Source: CAD feature listing. Evaluate the final solid. Frame: model axes, mm. A direction names the side the tool comes from. Round coordinates to 2 decimals unless told otherwise and drop trailing zeros. Order: outer loops, then holes, each group sorted by start corner. A loop starts at its lowest first (then second) coordinate and runs counter-clockwise, first axis right, second up.
Autodesk Inventor part; units mm, degrees
ref_plane "YZ Plane" through (0, 0, 0) normal (1, 0, 0) x (0, 1, 0)
ref_plane "XZ Plane" through (0, 0, 0) normal (0, 1, 0) x (-1, 0, 0)
ref_plane "XY Plane" through (0, 0, 0) normal (0, 0, 1) x (1, 0, 0)
sketch "Sketch1" plane through (0, 0, 0) normal (0, 1, 0) x (-1, 0, 0)
  line L0 (100, -50) -> (-100, -50)
  line L1 (-100, -50) -> (-100, 50)
  line L2 (-100, 50) -> (100, 50)
  line L3 (100, 50) -> (100, -50)
  line L4 (100, -50) -> (-100, 50) construction
  line L5 (-100, -50) -> (100, 50) construction
  line L6 (-40, -30) -> (-80, -30)
  line L7 (-50, -50) -> (-70, -50)
  line L8 (-40, -30) -> (-50, -50)
  line L9 (-80, -30) -> (-70, -50)
  line L10 (80, -30) -> (40, -30)
  line L11 (70, -50) -> (50, -50)
  line L12 (80, -30) -> (70, -50)
  line L13 (40, -30) -> (50, -50)
  line L14 (-100, -10) -> (-100, 10)
  line L15 (-80, -20) -> (-80, 20)
  line L16 (-80, -20) -> (-100, -10)
  line L17 (-80, 20) -> (-100, 10)
  line L18 (100, -50) -> (-100, -50)
  line L19 (-100, -50) -> (-100, -80)
  line L20 (-100, -80) -> (100, -80)
  line L21 (100, -80) -> (100, -50)
  line L22 (-40, -70) -> (-80, -70)
  line L23 (-40, -70) -> (-50, -50)
  line L24 (-80, -70) -> (-70, -50)
  line L25 (80, -70) -> (40, -70)
  line L26 (80, -70) -> (70, -50)
  line L27 (40, -70) -> (50, -50)
  line L28 (-100, -80) -> (-200, -80)
  line L29 (-200, -80) -> (-200, -50)
  line L30 (-200, -50) -> (-100, -50)
  line L31 (-100, -50) -> (-100, -80)
  line L32 (-160, -70) -> (-150, -50)
  line L33 (-160, -70) -> (-120, -70)
  line L34 (-120, -70) -> (-130, -50)
  line L35 (0, -80) -> (0, -50)
  point P0 (0, 0)
  point P1 (-100, 10)
  point P2 (-100, -10)
  point P3 (-70, -50)
  point P4 (-50, -50)
  point P5 (70, -50)
  point P6 (0, 0)
  point P7 (0, 0)
  point P8 (-100, -50)
  point P9 (-100, -50)
  point P10 (-100, -50)
  dimension "d72" = 200
  dimension "d73" = 100
  dimension "d78" = 20
  dimension "d79" = 40
  dimension "d80" = 20
  dimension "d81" = 10
  dimension "d82" = 20
  dimension "d83" = 40
  dimension "d84" = 20
  dimension "d85" = 10
  dimension "d86" = 120
  dimension "d87" = 30
  dimension "d88" = 0
  dimension "d89" = 0
  dimension "d90" = 40
  dimension "d91" = 20
  dimension "d92" = 20
  dimension "d93" = 10
  dimension "d94" = 40
  dimension "d95" = 0
  dimension "d114" = 200
  dimension "d115" = 30
  dimension "d128" = 100
sketch "Sketch1 outline for Extrusion28" plane through (0, 0, 0) normal (0, 1, 0) x (-1, 0, 0)
  line L0 (-200, -50) -> (-200, -80)
  line L1 (-100, -50) -> (-200, -50)
  line L2 (-100, -80) -> (-100, -50)
  line L3 (-200, -80) -> (-100, -80)
extrude "Extrusion28" add sketch "Sketch1 outline for Extrusion28" along normal blind 12
sketch "Sketch1 outline for Extrusion29" plane through (0, 0, 0) normal (0, 1, 0) x (-1, 0, 0)
  line L0 (-160, -70) -> (-120, -70)
  line L1 (-150, -50) -> (-160, -70)
  line L2 (-130, -50) -> (-150, -50)
  line L3 (-120, -70) -> (-130, -50)
extrude "Extrusion29" cut sketch "Sketch1 outline for Extrusion29" along normal blind 6
fillet "Fillet17" radius 6 2 edges at (150, 0, -80) (150, 12, -80)
fillet "Fillet18" radius 2 2 edges at (120, 3, -70) (160, 3, -70)
fillet "Fillet19" radius 1 5 edges at (158.4652, 0, -69.0515) (140, 0, -70) (121.5348, 0, -69.0515) (125.7236, 0, -58.5528) (154.2764, 0, -58.5528)
mirror "Mirror1" about plane through (100, 0, -80) normal (-1, 0, 0) of "Extrusion28", "Fillet17", "Extrusion29", "Fillet18", "Fillet19"
properties part number "Test2_3DPrint"
1. Pull-direction query (X, two-part tool) for faces 1 (the face through (200, 6, -65)), 2 (the face through (154.472, 0.301, -58.306)), 3 (the face through (101, 0, -62)); classes: released by +X, released by -X, zero draft, split by the parting line, or undercut.
2. First-contact query: pin 1 (2.5 mm diameter, centred on x = 136.5, y = 3.5, fed in from +Z); pin 2 (10 mm diameter, centred on x = 145, z = -60.5, fed in from -Y). Flat tips, straight axial feed; report the tip coordinate or a pass-through.
3. Access query for faces 4 (the face through (0, 6, -65)), 5 (the face through (60, 6, -62)). Directions: +Z, -Z, +X, -X, +Y, -Y. A direction counts if a zero-diameter tool reaches every point of the face in a straight line with its end or side. Return the directions, or none.
4. Section B-B on y = 3. Return loops of the section in (x, z), plus the area to 3 significant figures.
5. Line query: line 1 along X through (y, z) = (5, -63.5); line 2 along X through (y, z) = (3.5, -68); line 3 along Y through (x, z) = (59, -57.5). Output: solid intervals per line, ascending.
Result:
1. face 1: released by +X
1. face 2: undercut
1. face 3: zero draft
2. pin 1: stops at z = -70
2. pin 2: stops at y = 6
3. face 4: +Z, -Z, -X, +Y, -Y
3. face 5: -Y
4. outline: (0, -79.2) - (200, -79.2) - (200, -50) - (150, -50) - (158.55, -67.11) arc R2 cw to (156.76, -70) - (123.24, -70) arc R2 cw to (121.45, -67.11) - (130, -50) - (70, -50) - (78.55, -67.11) arc R2 cw to (76.76, -70) - (43.24, -70) arc R2 cw to (41.45, -67.11) - (50, -50) - (0, -50) - close
4. area: 4,650 mm2
5. line 1: x = 0 to 43.25, 76.75 to 123.25, 156.75 to 200
5. line 2: x = 0 to 41.24, 78.76 to 121.24, 158.76 to 200
5. line 3: y = 6 to 12
